```python
from build123d import *

# Parameters (mm, degrees)
F1_DEPTH = 6.35
F0_W     = 88.9
F0_H     = 26.67
F2_DEPTH = 127
F4_DEPTH = 6.35


with BuildPart() as f1:
    # F0 (on Top) → F1 (new body)
    with BuildSketch(Plane.XY):
        Polygon((38.1, -6.985), (38.1, 6.985), (-38.1, 6.985), (-38.1, -6.985), (-7.62, -6.985), (-7.62, 0), (7.62, 0), (7.62, -6.985), align=None)
    extrude(amount=F1_DEPTH)

    # F0 (on Top) → F2 (join)
    with BuildSketch(Plane.XY):
        Rectangle(F0_W, F0_H)
        Polygon((-38.1, 6.985), (38.1, 6.985), (38.1, -6.985), (7.62, -6.985), (-7.62, -6.985), (-38.1, -6.985), align=None, mode=Mode.SUBTRACT)
    extrude(amount=F2_DEPTH)

    # F3 (on face) → F4 (cut, through all)
    with BuildSketch(Plane.XZ.offset(13.335)):
        with BuildLine():
            Line((31.75, 127), (-31.75, 127))
            Line((-31.75, 127), (-31.75, 16.0443484783))
            Line((-31.75, 16.0443484783), (-8.9978614884, 16.0443484783))
            ThreePointArc((-8.9978614884, 16.0443484783), (0, 25.0422099667), (8.9978614884, 16.0443484783))
            Line((8.9978614884, 16.0443484783), (31.75, 16.0443484783))
            Line((31.75, 16.0443484783), (31.75, 127))
        make_face()
        with BuildLine():
            ThreePointArc((8.9978614884, 16.0443484783), (0, 25.0422099667), (-8.9978614884, 16.0443484783))
            Line((-8.9978614884, 16.0443484783), (8.9978614884, 16.0443484783))
        make_face()
        with BuildLine():
            Line((8.9978614884, 16.0443484783), (-8.9978614884, 16.0443484783))
            ThreePointArc((-8.9978614884, 16.0443484783), (0, 7.0464869899), (8.9978614884, 16.0443484783))
        make_face()
    extrude(amount=-F4_DEPTH, mode=Mode.SUBTRACT)


solid = f1.part
```
Read the model definition and answer for the solid it produces. Units are mm, in the model's axes. A direction names the side the tool comes from. Give positions to 0.01 mm unless a question says otherwise; leave off trailing zeros. Order: outer loops, then holes, each group sorted by start corner. A loop starts at its lowest first (then second) coordinate and runs counter-clockwise, first axis right, second up.
(1) Find section D-D (z = 51). Give the vertices of the cut face in (x, y) (3 decimals), plus the area to 3 significant figures.
(2) Find section B-B (x = 0). Give the vertices of the cut face in (y, z) (3 decimals), plus the area to 3 significant figures.
(3) Find section C-C (x = -36). Give the vertices of the cut face in (y, z) (3 decimals).
(4) Find section A-A (y = -2.75). Give the vertices of the cut face in (x, z).
(5) For faces 1 (the flat face through (-1, 6.985, 66)), 2 (the flat face through (20, -10, 16.044)), 3 (the flat face through (7.62, -3, 3)), 4 (the flat face through (-33, -13.335, 54)), determine the directions among +Z, -Z, +X, -X, +Y, -Y from which every point of the face is accessible in a straight line to the end or side of a thin tool.
(6) Straight lines are drawn through the part: L1, parallel to X at y = -0.75, z = 93.5; L2, parallel to X at y = -8, z = 82; L3, parallel to Y at x = -4.5, z = 7 (3 decimals). For each, find the intervals that lie inside material, in ascending order.
(7) Given pin 1 (7 mm diameter, centred on x = -21, y = -11.5, fed in from +Z); pin 2 (6 mm diameter, centred on x = -16.5, z = 50, fed in from -Y) (3 decimals); pin 3 (10 mm diameter, centred on x = -14.5, y = 6, fed in from +Z); pin 4 (4 mm diameter, centred on x = -15.5, y = -0.5, fed in from +Z), each flat-ended and moving along its own axis, determine where each tip first touches the part or whether it passes through.
(8) For a pull along X with two mould halves and no side action, classify faces 5 (the flat face through (-1, 2, 6.35)), 6 (the flat face through (0, 0, 3)), 7 (the flat face through (-44.45, 0, 63)), 8 (the flat face through (44.45, 0, 63)) as released by +X, released by -X, zero draft, split by the parting line, or undercut.
Result sheet:
1. outline: (-44.45, -13.335) - (-31.75, -13.335) - (-31.75, -6.985) - (-38.1, -6.985) - (-38.1, 6.985) - (38.1, 6.985) - (38.1, -6.985) - (31.75, -6.985) - (31.75, -13.335) - (44.45, -13.335) - (44.45, 13.335) - (-44.45, 13.335) - close
1. area: 903 mm2
2. outline: (-13.335, 0) - (-6.985, 0) - (-6.985, 7.046) - (-13.335, 7.046) - close; (0, 0) - (13.335, 0) - (13.335, 127) - (6.985, 127) - (6.985, 6.35) - (0, 6.35) - close
2. area: 896 mm2
3. outline: (-13.335, 0) - (13.335, 0) - (13.335, 127) - (6.985, 127) - (6.985, 6.35) - (-6.985, 6.35) - (-6.985, 127) - (-13.335, 127) - close
4. outline: (-44.45, 0) - (-7.62, 0) - (-7.62, 6.35) - (-38.1, 6.35) - (-38.1, 127) - (-44.45, 127) - close; (7.62, 0) - (44.45, 0) - (44.45, 127) - (38.1, 127) - (38.1, 6.35) - (7.62, 6.35) - close
5. face 1: +Z
5. face 2: +Z, -Y
5. face 3: +Z, -Z
5. face 4: +Z, -Z, +X, -X, -Y
6. L1: x = -44.45 to -38.1, 38.1 to 44.45
6. L2: x = -44.45 to -31.75, 31.75 to 44.45
6. L3: y = -13.335 to -6.985, 6.985 to 13.335
7. pin 1: stops at z = 16.04
7. pin 2: stops at y = 6.985
7. pin 3: stops at z = 127
7. pin 4: stops at z = 6.35
8. face 5: undercut
8. face 6: undercut
8. face 7: released by -X
8. face 8: released by +X
